Job drawing, mm, ordinate dimensions from the low corner. One solid piece. A direction names the side the tool comes from. Give positions to 0.01 mm unless a question says otherwise; leave off trailing zeros. Order: outer loops, then holes, each group sorted by start corner. A loop starts at its lowest first (then second) coordinate and runs counter-clockwise, first axis right, second up. Notation, with made-up numbers: (8, 13.5) - (14, 13.5) arc R5 ccw to (14, 21.5) - close; hole circle Ø11 at (72, 66). An arc over 180 degrees is marked (long way). Use a Markdown table: item, result. Add a question column.
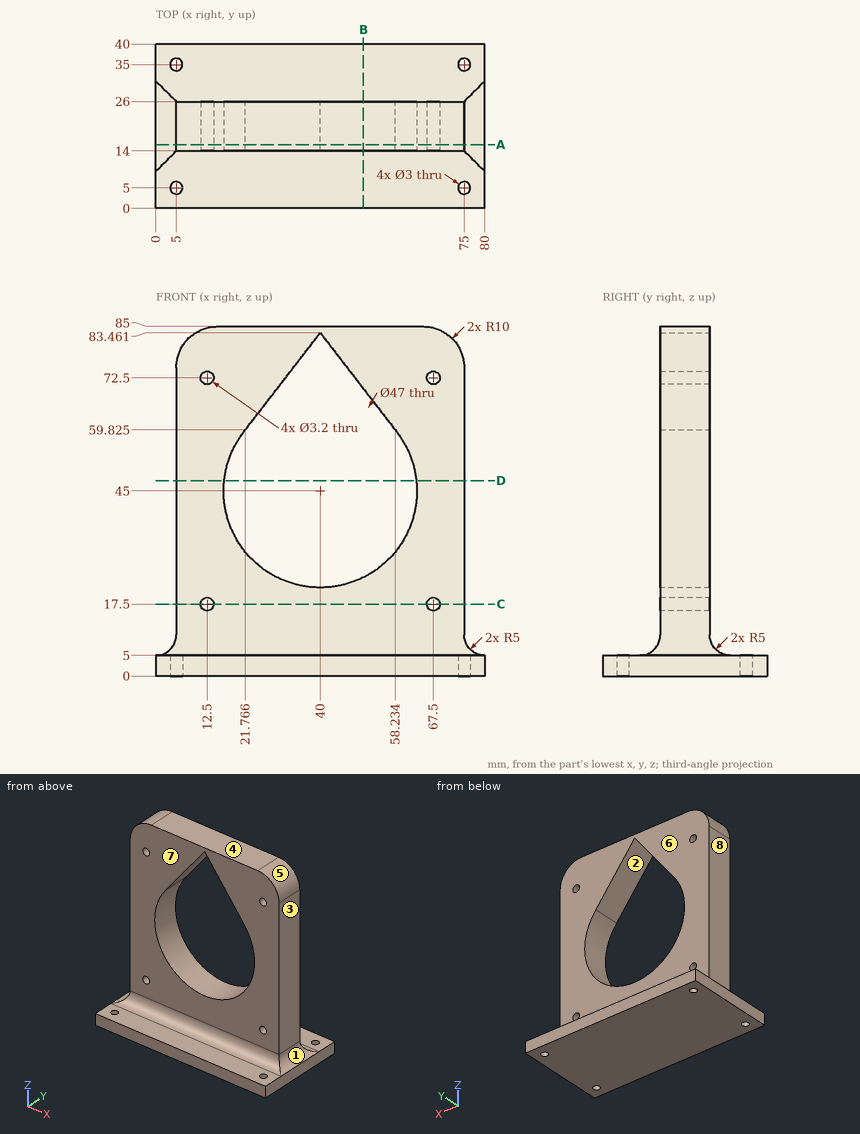
1. Tool access for the marked faces 4, 5, 6, 7 and 8: list every direction of +Z, -Z, +X, -X, +Y, -Y with a clear straight run to the whole face (end or side of a thin tool).
2. Pin check, flat tips, straight feed: P1, Ø3.5, axis at x = 67.5, z = 17.5, coming from the -Y side; P2, Ø8, axis at y = 28, z = 40, coming from the -X side; P3, Ø8, axis at x = 11, z = 12.5, coming from the -Y side. Stop position of each tip, or through.
3. Mould opens along Z. For the marked faces 1, 2 and 3 say: released by +Z, released by -Z, zero draft, split by the parting line, or undercut.
4. Cut at D-D (z = 47.5). Write the cut outline in (x, y).
5. Cut at B-B (x = 50.5). Write the cut outline in (y, z), plus the area to 3 significant figures.
6. Cut at A-A (y = 15.5). State how many separate pieces and enclosed holes the cut face has, plus the area to 3 significant figures.
7. Cut at C-C (z = 17.5). Write the cut outline in (x, y).
8. Drill centre lines: probe 1 along X at (y, z) = (17.25, 17.5); probe 2 along Y at (x, z) = (75, 3.45); probe 3 along Z at (x, y) = (67.5, 21.25). Where is each one in solid material? Low to high. Write a range as [from, to].
Responses:
| question | item | result |
|---|---|---|
| 1 | face 4 | +Z, +X, -X, +Y, -Y |
| 1 | face 5 | +Z, +X, +Y, -Y |
| 1 | face 6 | +Z, +X, -X, +Y |
| 1 | face 7 | +Z, +X, -X, -Y |
| 1 | face 8 | +Z, -X, +Y, -Y |
| 2 | P1 | stops at y = 14 |
| 2 | P2 | stops at x = 5 |
| 2 | P3 | stops at y = 13.77 |
| 3 | face 1 | released by +Z |
| 3 | face 2 | undercut |
| 3 | face 3 | zero draft |
| 4 | outline | (5, 14) - (16.63, 14) - (16.63, 26) - (5, 26) - close; (63.37, 14) - (75, 14) - (75, 26) - (63.37, 26) - close |
| 5 | outline | (0, 0) - (40, 0) - (40, 5) - (31, 5) arc R5 cw to (26, 10) - (26, 23.98) - (14, 23.98) - (14, 10) arc R5 cw to (9, 5) - (0, 5) - close; (14, 69.85) - (26, 69.85) - (26, 85) - (14, 85) - close |
| 5 | area | 620 mm² |
| 6 | separate pieces | 1 |
| 6 | enclosed holes | 5 |
| 6 | area | 3,990 mm² |
| 7 | outline | (5, 14) - (10.9, 14) - (10.9, 26) - (5, 26) - close; (14.1, 14) - (65.9, 14) - (65.9, 26) - (14.1, 26) - close; (69.1, 14) - (75, 14) - (75, 26) - (69.1, 26) - close |
| 8 | probe 1 | x = [5, 10.9], [14.1, 65.9], [69.1, 75] |
| 8 | probe 2 | y = [0, 3.5], [6.5, 33.5], [36.5, 40] |
| 8 | probe 3 | z = [0, 15.9], [19.1, 70.9], [74.1, 84.68] |
